Geometry check sheet. Reference: the model listing, model coordinates, mm. Face numbers are marked on the shaded views. A direction names the side the tool comes from. Give positions to 0.01 mm unless a question says otherwise; leave off trailing zeros. Loops run counter-clockwise (first coordinate to the right, second up) from the corner with the lowest first, then second, coordinate; pieces in that order, holes last. Notation, with made-up numbers: (83, 35.5) - (113, 35.5) arc R15 ccw to (113, 45.5) - close; hole circle Ø6 at (61.5, 12.5). An arc over 180 degrees is marked (long way). Use a Markdown table: item, result. Add a question column.
1. Depth check by flat-ended pin: P1, Ø7.5, axis at x = 3.5, y = 27, coming from the -Z side; P2, Ø6, axis at y = 44, z = -29.5, coming from the +X side; P3, Ø4, axis at y = 33.5, z = -23, coming from the -X side (3 decimals). Enter the tip coordinate at first touch or a pass-through.
2. Set-up check for the marked faces 1, 2, 3, 4 and 5: record each of +Z, -Z, +X, -X, +Y, -Y from which the full face is reachable in a straight line by a thin tool's end or side.
3. Cross-section at D-D on z = -38. Enter the section's corners in (x, y).
4. Material ranges on L1, parallel to Z at x = 19.05, y = 39 (1 decimal); L2, parallel to Z at x = 19.05, y = 25.5 (1 decimal); L3, parallel to X at y = 43, z = -21 (3 decimals), recorded low to high.
5. Cross-section at C-C on x = 19.05. Enter the section's corners in (y, z) (1 decimal), and give its area (3 significant figures).
6. Cross-section at B-B on x = 8.5. Enter the section's corners in (y, z).
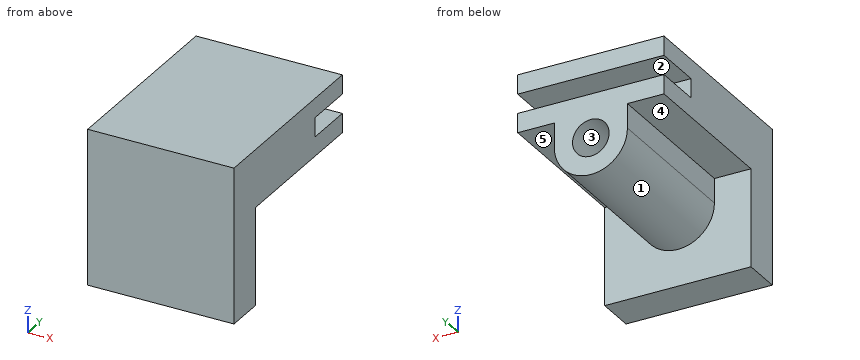
from build123d import *

# Parameters (mm, degrees)
BOSS_EXTRUDE1_DEPTH = 38.1
BOSS_EXTRUDE2_REACH = 52.8
SKETCH2_R           = 4.7625


with BuildPart() as part:
    # Sketch1 → Boss-Extrude1 (new body)
    with BuildSketch(Plane(origin=(0, 0, 0), x_dir=(0, 0, -1), z_dir=(1, 0, 0))):
        Polygon((0, 0), (40.4, 0), (40.4, 10), (15, 10), (15, 50.8), (10, 50.8), (10, 38.1), (5, 38.1), (5, 50.8), (0, 50.8), align=None)
    extrude(amount=BOSS_EXTRUDE1_DEPTH)

    # Sketch2 → Boss-Extrude2 (add, up to next)
    with BuildSketch(Plane(origin=(0, 50.8, 0), x_dir=(1, 0, 0), z_dir=(0, 1, 0)), mode=Mode.PRIVATE) as boss_extrude2_sk1:
        with BuildLine():
            Line((9.525, 21.35), (9.525, 15))
            Line((9.525, 15), (28.575, 15))
            Line((28.575, 15), (28.575, 21.35))
            ThreePointArc((28.575, 21.35), (19.05, 30.875), (9.525, 21.35))
        make_face()
        with Locations((19.05, 21.35)):
            Circle(SKETCH2_R, mode=Mode.SUBTRACT)
    boss_extrude2_tool1 = extrude(boss_extrude2_sk1.sketch, amount=-BOSS_EXTRUDE2_REACH, mode=Mode.PRIVATE) - part.part
    add(boss_extrude2_tool1.solids().sort_by_distance((9.772975, 50.8, -18.175))[0])


solid = part.part
Values found:
| question | item | result |
|---|---|---|
| 1 | P1 | stops at z = -15 |
| 1 | P2 | stops at x = 27.06 |
| 1 | P3 | stops at x = 9.525 |
| 2 | face 1 | -Z, +Y |
| 2 | face 2 | +X, -X, +Y |
| 2 | face 3 | +Y |
| 2 | face 4 | -Z, -X, +Y |
| 2 | face 5 | -Z, +X, +Y |
| 3 | outline | (0, 0) - (38.1, 0) - (38.1, 10) - (0, 10) - close |
| 4 | L1 | z = -30.9 to -26.1, -16.6 to -10, -5 to 0 |
| 4 | L2 | z = -30.9 to -26.1, -16.6 to 0 |
| 4 | L3 | x = 9.525 to 14.3, 23.8 to 28.575 |
| 5 | outline | (0, -40.4) - (10, -40.4) - (10, -30.9) - (50.8, -30.9) - (50.8, -26.1) - (10, -26.1) - (10, -16.6) - (50.8, -16.6) - (50.8, -10) - (38.1, -10) - (38.1, -5) - (50.8, -5) - (50.8, 0) - (0, 0) - close |
| 5 | area | 1,210 mm2 |
| 6 | outline | (0, -40.4) - (10, -40.4) - (10, -15) - (50.8, -15) - (50.8, -10) - (38.1, -10) - (38.1, -5) - (50.8, -5) - (50.8, 0) - (0, 0) - close |
